```python
from build123d import *

# Parameters (mm, degrees)
F1_DEPTH = 1866
F2_W     = 30
F2_H     = 30
F3_DEPTH = 880
F4_W     = 30
F4_H     = 30
F5_DEPTH = 550
F6_W     = 30
F6_H     = 30
F7_DEPTH = 100
F8_W     = 30
F8_H     = 30
F9_DEPTH = 1746


with BuildPart() as f1:
    # F0 (on Right) → F1 (new body)
    with BuildSketch(Plane.YZ):
        Polygon((0, 30), (0, 0), (740, 0), (740, 130), (720, 130), (720, 30), align=None)
    extrude(amount=F1_DEPTH)

    # F2 (on face) → F3 (join)
    with BuildSketch(Plane(origin=(0, 0, 0), x_dir=(1, 0, 0), z_dir=(0, 0, -1))):
        with Locations((45, -45)):
            Rectangle(F2_W, F2_H)
        with Locations((1821, -45)):
            Rectangle(F2_W, F2_H)
        with Locations((1821, -625)):
            Rectangle(F2_W, F2_H)
        with Locations((45, -625)):
            Rectangle(F2_W, F2_H)
    extrude(amount=F3_DEPTH)

    # F4 (on face) → F5 (join, through all)
    with BuildSketch(Plane.XZ.offset(-610)):
        with Locations((45, -715)):
            Rectangle(F4_W, F4_H)
        with Locations((1821, -715)):
            Rectangle(F4_W, F4_H)
    extrude(amount=F5_DEPTH)

    # F6 (on face) → F7 (join)
    with BuildSketch(Plane(origin=(0, 640, 0), x_dir=(-1, 0, 0), z_dir=(0, 1, 0))):
        with Locations((-45, -440)):
            Rectangle(F6_W, F6_H)
        with Locations((-1821, -440)):
            Rectangle(F6_W, F6_H)
    extrude(amount=F7_DEPTH)

    # F8 (on face) → F9 (join, through all)
    with BuildSketch(Plane.YZ.offset(60)):
        with Locations((725, -440)):
            Rectangle(F8_W, F8_H)
    extrude(amount=F9_DEPTH)


solid = f1.part
```
Can you work these out from the model? Positions are in its coordinate system, mm. A direction names the side the tool comes from. Coordinates: 2 decimals unless noted, no trailing zeros. Loops run counter-clockwise (first coordinate to the right, second up) from the corner with the lowest first, then second, coordinate; pieces in that order, holes last. Notation, with made-up numbers: (50, 20) -> (76, 20) arc R23 ccw to (76, 45) -> close; hole circle Ø7 at (-26.75, 87). An arc over 180 degrees is marked (long way). Put each result on its own line as item: value. Start each with the question number.
Q1. I want a section at C-C (x = 416). Write out the boundary of the cut face in (y, z), plus the area to 3 significant figures.
Q2. I'm going to push flat-ended pins straight in: P1, Ø24, axis at x = 47.5, z = -235, coming from the -Y side; P2, Ø9, axis at x = 1824, z = -820, coming from the +Y side; P3, Ø4, axis at x = 1502.5, y = 646, coming from the -Z side. Where does each tip first touch, or does it pass through?
Q3. I want a section at B-B (y = 327). Write out the boundary of the cut face in (x, z).
Q4. I want a section at A-A (z = -187). Write out the boundary of the cut face in (x, y), plus the area to 3 significant figures.
Q5. For faces 4 (the face through (1836, 623, -438)), 5 (the face through (862, 716, -455)), 6 (the face through (30, 623, -438)), 7 (the face through (920, 720, 81)), which set-ups out of +Z, -Z, +X, -X, +Y, -Y let a thin tool reach every point of the face, with its end or its side?
Q6. If I drill on line 1 (X direction, y = 37, z = -440); line 2 (Z direction, x = 1367, y = 485); line 3 (Y direction, x = 622, z = 71), over which ranges is the centre line in solid material (lowest first)? Write a range as [from, to].
Q7. Thinking about a two-plate mould opening in Z: for faces 1 (the face through (920, 365, 30)), 2 (the face through (862, 716, -425)), 3 (the face through (1866, 396, 17)), which applies, pulls with the +Z half, pulls with the -Z half, needs draft (parallel to the pull), parting line crosses it, or undercut?
Taken from the geometry:
1. outline: (0, 0) -> (740, 0) -> (740, 130) -> (720, 130) -> (720, 30) -> (0, 30) -> close; (710, -455) -> (740, -455) -> (740, -425) -> (710, -425) -> close
1. area: 25,100 mm2
2. P1: stops at y = 30
2. P2: stops at y = 640
2. P3: stops at z = 0
3. outline: (0, 0) -> (1866, 0) -> (1866, 30) -> (0, 30) -> close; (30, -730) -> (60, -730) -> (60, -700) -> (30, -700) -> close; (1806, -730) -> (1836, -730) -> (1836, -700) -> (1806, -700) -> close
4. outline: (30, 30) -> (60, 30) -> (60, 60) -> (30, 60) -> close; (30, 610) -> (60, 610) -> (60, 640) -> (30, 640) -> close; (1806, 30) -> (1836, 30) -> (1836, 60) -> (1806, 60) -> close; (1806, 610) -> (1836, 610) -> (1836, 640) -> (1806, 640) -> close
4. area: 3,600 mm2
5. face 4: -Z, +X, +Y, -Y
5. face 5: -Z, +X, -X, +Y
5. face 6: -Z, -X, +Y, -Y
5. face 7: +Z, +X, -X, -Y
6. line 1: x = [30, 60], [1806, 1836]
6. line 2: z = [0, 30]
6. line 3: y = [720, 740]
7. face 1: pulls with the +Z half
7. face 2: undercut
7. face 3: needs draft
